```python
from build123d import *

# Parameters (mm, degrees)
CROQUIS1_W               = 65
CROQUIS1_H               = 146
SALIENTE_EXTRUIR1_DEPTH  = 3
CROQUIS2_W               = 8
CROQUIS2_H               = 3
SALIENTE_EXTRUIR2_DEPTH  = 5
REDONDEO1_R              = 4
REDONDEO1_OF_SIMETR_A1_R = 4
CROQUIS3_W               = 2.60095456
CROQUIS3_H               = 3.001101416
SALIENTE_EXTRUIR3_DEPTH  = 0.8
REDONDEO2_R              = 2
REDONDEO2_OF_SIMETR_A5_R = 2
CROQUIS4_W               = 65
CROQUIS4_H               = 3
CROQUIS4_W_2             = 30
CROQUIS4_H_2             = 2
SALIENTE_EXTRUIR4_DEPTH  = 3
REDONDEO3_R              = 60
CROQUIS6_W               = 3.139643751
CROQUIS6_H               = 2.781946526
CORTAR_EXTRUIR1_DEPTH    = 10
CROQUIS8_R               = 1.75
CORTAR_EXTRUIR2_DEPTH    = 10


# Some blends are built 0.0001 mm under size
with BuildPart() as part:
    # Croquis1 → Saliente-Extruir1 (new body)
    with BuildSketch(Plane(origin=(0, 0, 0), x_dir=(1, 0, 0), z_dir=(0, 1, 0))):
        Rectangle(CROQUIS1_W, CROQUIS1_H)
    extrude(amount=SALIENTE_EXTRUIR1_DEPTH)

    # Croquis2 → Saliente-Extruir2 (add)
    with BuildSketch(Plane(origin=(32.5, 0, 0), x_dir=(0, 0, -1), z_dir=(1, 0, 0))):
        with Locations((66, 1.5)):
            Rectangle(CROQUIS2_W, CROQUIS2_H)
    saliente_extruir2 = extrude(amount=SALIENTE_EXTRUIR2_DEPTH)

    # Redondeo1
    redondeo1_edges = [part.edges().sort_by_distance(p)[0] for p in [
        (37.5, 1.5, -62),
        (37.5, 1.5, -70),
    ]]
    fillet(redondeo1_edges, radius=REDONDEO1_R - 0.0001)  # a hair under: the kernel refuses the full size

    # Simetría1: Saliente-Extruir2 across plane
    add(saliente_extruir2.mirror(Plane(origin=(0, 0, 0), x_dir=(0, 0, 1), z_dir=(1, 0, 0))))

    # Redondeo1 of Simetría1
    redondeo1_of_simetr_a1_edges = [part.edges().sort_by_distance(p)[0] for p in [
        (-37.5, 1.5, -62),
        (-37.5, 1.5, -70),
    ]]
    fillet(redondeo1_of_simetr_a1_edges, radius=REDONDEO1_OF_SIMETR_A1_R - 0.0001)  # a hair under: the kernel refuses the full size

    # Croquis3 → Saliente-Extruir3 (add)
    with BuildSketch(Plane(origin=(32.5, 0, 0), x_dir=(0, 0, -1), z_dir=(1, 0, 0))):
        with Locations((-53.003039433, 1.500550708)):
            Rectangle(CROQUIS3_W, CROQUIS3_H)
    saliente_extruir3 = extrude(amount=SALIENTE_EXTRUIR3_DEPTH)

    # Redondeo2
    # the kernel refuses this fillet: 2 mm, written as the material it takes off along each edge
    with BuildSketch(Plane(origin=(33.3, 7.001101416, 51.702562153), x_dir=(-1, 0, 0), z_dir=(0, -1, 0)), Plane(origin=(33.3, -4, 54.303516713), x_dir=(-1, 0, 0), z_dir=(0, 1, 0))) as redondeo2_piece_1:
        with BuildLine():
            CenterArc((2, -1.6), REDONDEO2_R, 126.869897646, 53.130102354)
            Line((0, -1.6), (-0.04, -1.6))
            Line((-0.04, -1.6), (-0.04, 0))
            Line((-0.04, 0), (0, 0.04))
            ThreePointArc((0, 0.04), (0.4, 0.04), (0.776, 0.032))
            Line((0.776, 0.032), (0.8, 0))
        make_face()
    extrude(amount=11.001101416, mode=Mode.SUBTRACT)

    # Simetría5: Saliente-Extruir3 across plane
    add(saliente_extruir3.mirror(Plane(origin=(0, 0, 0), x_dir=(0, 0, 1), z_dir=(1, 0, 0))))

    # Redondeo2 of Simetría5
    # the kernel refuses this fillet: 2 mm, written as the material it takes off along each edge
    with BuildSketch(Plane(origin=(-33.3, 7.001101416, 51.702562153), x_dir=(1, 0, 0), z_dir=(0, -1, 0)), Plane(origin=(-33.3, -4, 54.303516713), x_dir=(1, 0, 0), z_dir=(0, 1, 0))) as redondeo2_of_simetr_a5_piece_1:
        with BuildLine():
            CenterArc((2, 1.6), REDONDEO2_OF_SIMETR_A5_R, 180, 53.130102354)
            Line((0, 1.6), (-0.04, 1.6))
            Line((-0.04, 1.6), (-0.04, 0))
            Line((-0.04, 0), (0, -0.04))
            ThreePointArc((0, -0.04), (0.4, -0.04), (0.776, -0.032))
            Line((0.776, -0.032), (0.8, 0))
        make_face()
    extrude(amount=11.001101416, mode=Mode.SUBTRACT)

    # Croquis4 → Saliente-Extruir4 (add)
    with BuildSketch(Plane(origin=(0, 3, 0), x_dir=(1, 0, 0), z_dir=(0, 1, 0))):
        with Locations((0, -74.5)):
            Rectangle(CROQUIS4_W, CROQUIS4_H)
        with Locations((11.5, -77)):
            Rectangle(CROQUIS4_W_2, CROQUIS4_H_2)
    extrude(amount=-SALIENTE_EXTRUIR4_DEPTH)

    # Redondeo3
    # the kernel refuses this fillet: 60 mm, written as the material it takes off along each edge
    with BuildSketch(Plane(origin=(26.5, 41.405728739, 78), x_dir=(0, 0, -1), z_dir=(0, -1, 0))) as redondeo3_piece_1:
        with BuildLine():
            CenterArc((60, -15.362291496), REDONDEO3_R, 165.164888418, 14.835111582)
            Line((0, -15.362291496), (0, 0))
            Line((0, 0), (2, 0))
        make_face()
    extrude(amount=79.811457479, mode=Mode.SUBTRACT)
    with BuildSketch(Plane(origin=(-3.5, 41.405728739, 78), x_dir=(1, 0, 0), z_dir=(0, -1, 0))) as redondeo3_piece_2:
        with BuildLine():
            CenterArc((15.362291496, -60), REDONDEO3_R, 90, 14.835111582)
            Line((0, -2), (0, 0))
            Line((0, 0), (15.362291496, 0))
        make_face()
    extrude(amount=79.811457479, mode=Mode.SUBTRACT)

    # Croquis6 → Cortar-Extruir1 (cut)
    with BuildSketch(Plane(origin=(0, 3, 0), x_dir=(1, 0, 0), z_dir=(0, 1, 0))):
        with Locations((-30.930178125, 71.609026737)):
            Rectangle(CROQUIS6_W, CROQUIS6_H)
    extrude(amount=-CORTAR_EXTRUIR1_DEPTH, mode=Mode.SUBTRACT)

    # Croquis8 → Cortar-Extruir2 (cut)
    with BuildSketch(Plane(origin=(0, 3, 0), x_dir=(1, 0, 0), z_dir=(0, 1, 0))):
        with Locations(Location((11.5, -74.5, 0), (0, 0, 270))):
            Circle(CROQUIS8_R)
    extrude(amount=-CORTAR_EXTRUIR2_DEPTH, mode=Mode.SUBTRACT)


solid = part.part
```
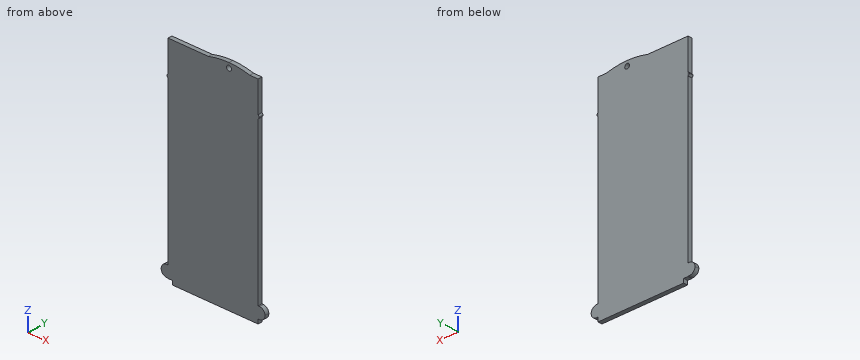
Input: part model. Units: mm. Frame: model coordinates. Coordinates: 2 decimals unless noted, no trailing zeros. Loops run counter-clockwise (first coordinate to the right, second up) from the corner with the lowest first, then second, coordinate; pieces in that order, holes last. Notation, with made-up numbers: (-33.75, -34.75) - (-1.75, -34.75) arc R3 ccw to (-1.75, -29.75) - close; hole circle Ø10 at (-2, -1). An arc over 180 degrees is marked (long way). Answer in a Markdown table with one row per item.
(1) Cut plane B-B on z = 74.5. Output: boundary loops of the cut face in (x, y).
Model answer:
| item | result |
|---|---|
| outline | (-32.5, 0) - (9.75, 0) - (9.75, 3) - (-32.5, 3) - close; (13.25, 0) - (32.5, 0) - (32.5, 3) - (13.25, 3) - close |
(2) Material intervals for L1, parallel to X at y = 0.7, z = 74.5; L2, parallel to Y at x = 3.5, z = -4; L3, parallel to X at y = 2.2, z = 56.5, sorted ascending. Write a range as from..to.
Model answer:
| item | result |
|---|---|
| L1 | x = -32.5..9.75, 13.25..32.5 |
| L2 | y = 0..3 |
| L3 | x = -32.5..32.5 |
(3) Pin query (flat end, axial travel): P1, Ø0.5, axis at x = -33, y = 1, coming from the -Z side; P2, Ø1.5, axis at x = -21.5, y = 1, coming from the +Z side; P3, Ø0.9, axis at y = 1, z = 70.5, coming from the -X side; P4, Ø3, axis at x = 11.5, z = 74.5, coming from the -Y side. Return the tip coordinate at first contact, or that it passes through.
Model answer:
| item | result |
|---|---|
| P1 | stops at z = -70 |
| P2 | stops at z = 76 |
| P3 | stops at x = -32.5 |
| P4 | passes through |
(4) Cut plane C-C on z = -43. Output: boundary loops of the cut face in (x, y), plus the area to 3 significant figures.
Model answer:
| item | result |
|---|---|
| outline | (-32.5, 0) - (32.5, 0) - (32.5, 3) - (-32.5, 3) - close |
| area | 195 mm² |
